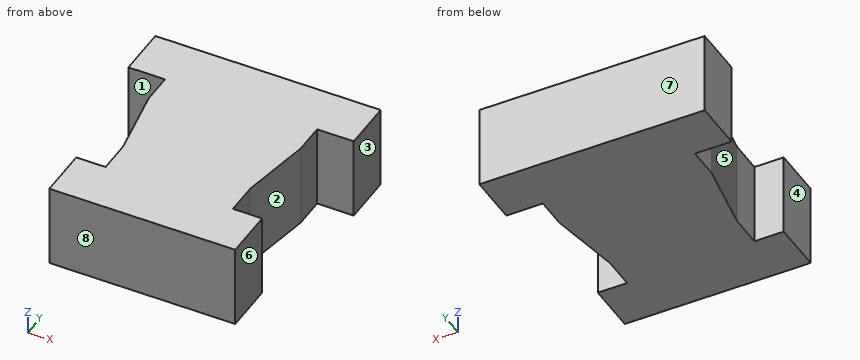
```python
from build123d import *

# Parameters (mm, degrees)
F0_W     = 40
F0_H     = 42
F1_DEPTH = 14.8
F3_DEPTH = 25


with BuildPart() as f1:
    # F0 (on Top) → F1 (new body)
    with BuildSketch(Plane.XY):
        Rectangle(F0_W, F0_H)
    extrude(amount=F1_DEPTH)

    # F2 (on face) → F3 (cut)
    with BuildSketch(Plane.XY.offset(14.8)):
        Polygon((-13.5, 12), (-20, 12), (-20, -21), (-16.5, -21), (-16.5, -12), (-11.3, -12), (-11.3, -6.2), (-13.5, 6.5), align=None)
        Polygon((16.5, -12), (16.5, -21), (20, -21), (20, 12), (13.5, 12), (13.5, 6.5), (11.3, -6.2), (11.3, -12), align=None)
    extrude(amount=-F3_DEPTH, mode=Mode.SUBTRACT)


solid = f1.part
```
Source: CAD feature listing. Evaluate the final solid. Frame: model axes, mm. Face numbers are marked on the shaded views. A direction names the side the tool comes from. Round coordinates to 2 decimals unless told otherwise and drop trailing zeros. Loops run counter-clockwise (first coordinate to the right, second up) from the corner with the lowest first, then second, coordinate; pieces in that order, holes last. Notation, with made-up numbers: M -35.75,-4 L -0.75,-4 A30 cw -0.75,26 Z; hole C 38.5,35 d6. An arc over 180 degrees is marked long. Use a Markdown table: item, result. Add a question column.
1. Line query: line 1 (Y direction, x = -16, z = 6); line 2 (X direction, y = -17, z = 8.5); line 3 (X direction, y = 7, z = 10). Output: solid intervals per line, ascending.
2. Section query D-D on y = -5.5. Return the cut outline in (x, z), then the cut area to 3 significant figures.
3. Contact query for flat-ended pins moving along their axis: P1, Ø1.5, axis at y = -14.5, z = 4, coming from the +X side; P2, Ø6, axis at y = -16.5, z = 13, coming from the -X side; P3, Ø3, axis at y = 8, z = 9, coming from the +X side. Output: stop coordinate, or through.
4. Mould query, pull axis Y, two halves, no side actions, for the marked faces 5, 6, 7 and 8. Classes: pulls with the +Y half, pulls with the -Y half, needs draft (parallel to the pull), parting line crosses it, or undercut.
5. Reachability of the marked faces 1, 2, 3 and 4 from +Z, -Z, +X, -X, +Y, -Y: full face, straight path, thin tool, end or side. Return the list, or none.
6. Section query C-C on y = 8. Return the cut outline in (x, z), then the cut area to 3 significant figures.
7. Section query B-B on z = 11.5. Return the cut outline in (x, y).
8. Section query A-A on x = 16. Return the cut outline in (y, z).
Reported:
| question | item | result |
|---|---|---|
| 1 | line 1 | y = -21 to -12, 12 to 21 |
| 1 | line 2 | x = -16.5 to 16.5 |
| 1 | line 3 | x = -13.5 to 13.5 |
| 2 | outline | M -11.42,0 L 11.42,0 L 11.42,14.8 L -11.42,14.8 Z |
| 2 | area | 338 mm² |
| 3 | P1 | stops at x = 16.5 |
| 3 | P2 | stops at x = -16.5 |
| 3 | P3 | stops at x = 13.5 |
| 4 | face 5 | undercut |
| 4 | face 6 | needs draft |
| 4 | face 7 | pulls with the +Y half |
| 4 | face 8 | pulls with the -Y half |
| 5 | face 1 | +Z, -Z, -X |
| 5 | face 2 | +Z, -Z, +X |
| 5 | face 3 | +Z, -Z, +X, +Y, -Y |
| 5 | face 4 | +Z, -Z, -X, -Y |
| 6 | outline | M -13.5,0 L 13.5,0 L 13.5,14.8 L -13.5,14.8 Z |
| 6 | area | 400 mm² |
| 7 | outline | M -20,12 L -13.5,12 L -13.5,6.5 L -11.3,-6.2 L -11.3,-12 L -16.5,-12 L -16.5,-21 L 16.5,-21 L 16.5,-12 L 11.3,-12 L 11.3,-6.2 L 13.5,6.5 L 13.5,12 L 20,12 L 20,21 L -20,21 Z |
| 8 | outline | M -21,0 L -12,0 L -12,14.8 L -21,14.8 Z; M 12,0 L 21,0 L 21,14.8 L 12,14.8 Z |
